Part model, mm, in its own coordinate system. Give positions to 0.01 mm unless a question says otherwise; leave off trailing zeros. Write each loop counter-clockwise with the first axis right and the second up, starting at its lowest first coordinate (ties: lowest second). Pieces come first, ordered by that corner, then holes. Notation, with made-up numbers: M -13,84.25 L 6,84.25 A18 ccw 6,109.25 Z; hole C 36.5,29.25 d4. An arc over 180 degrees is marked long. Use CSV: the item, a comma, the result in double quotes. Start each with the question number.
1. Mould opens along Z. For faces 1 (the face through (66.183, 1.479, 68.153)), 2 (the face through (57, 3, 57)), 3 (the face through (83.29, 1.48, 6.55)) say: pulls with the +Z half, pulls with the -Z half, needs draft (parallel to the pull), parting line crosses it, or undercut.
2. Band-saw the part on D-D, the plane y = 0.8. Count the separate pieces of the cut face and the enclosed holes in it, then the cut area to 3 significant figures.
3. Drop flat-ended pins along their axis: pin 1 Ø4 at (x, z) = (0, 89) entering from -Y; pin 2 Ø2 at (x, z) = (6.93, 85) entering from +Y; pin 3 Ø1.5 at (x, y) = (12, 1.5) entering from +Z; pin 4 Ø1.5 at (y, z) = (0.5, 67) entering from +X. Give the stop position or say it passes through.
4. Band-saw the part on B-B, the plane x = 0. List the corners of the cut face in (y, z), then the cut area to 3 significant figures.
5. Band-saw the part on A-A, the plane z = 0. List the corners of the cut face in (x, y), then the cut area to 3 significant figures.
6. Band-saw the part on C-C, the plane z = 89. List the corners of the cut face in (x, y), then the cut area to 3 significant figures.
7. Drill centre lines: line 1 along X through (y, z) = (0.9, 0); line 2 along Z through (x, y) = (-1, 2.7); line 3 along Z through (x, y) = (85, 1.1). Where is each one in solid material? Low to high. Write a range as from..to.
from build123d import *

# Parameters (mm, degrees)
SKETCH_1_R      = 1.75
EXTRUDE_1_DEPTH = 3


with BuildPart() as part:
    # 草图1 → 凸台-拉伸1 (new body)
    with BuildSketch(Plane(origin=(0, 0, 0), x_dir=(1, 0, 0), z_dir=(0, 1, 0))):
        with BuildLine():
            Line((-19.411428383, -72.444436972), (-24.587809285, -91.762953497))
            ThreePointArc((-24.587809285, -91.762953497), (67.175144213, -67.175144213), (91.762953497, 24.587809285))
            Line((91.762953497, 24.587809285), (72.444436972, 19.411428383))
            ThreePointArc((72.444436972, 19.411428383), (53.033008589, -53.033008589), (-19.411428383, -72.444436972))
        make_face()
        with Locations(Location((0, -89, 0), (0, 0, 270))):
            Circle(SKETCH_1_R, mode=Mode.SUBTRACT)
        with Locations(Location((0, -81, 0), (0, 0, 270))):
            Circle(SKETCH_1_R, mode=Mode.SUBTRACT)
        with Locations(Location((-6.92820323, -85, 0), (0, 0, 270))):
            Circle(SKETCH_1_R, mode=Mode.SUBTRACT)
        with Locations(Location((6.92820323, -85, 0), (0, 0, 270))):
            Circle(SKETCH_1_R, mode=Mode.SUBTRACT)
        with Locations(Location((85, -6.92820323, 0), (0, 0, 270))):
            Circle(SKETCH_1_R, mode=Mode.SUBTRACT)
        with Locations(Location((81, 0, 0), (0, 0, 270))):
            Circle(SKETCH_1_R, mode=Mode.SUBTRACT)
        with Locations(Location((85, 6.92820323, 0), (0, 0, 270))):
            Circle(SKETCH_1_R, mode=Mode.SUBTRACT)
        with Locations(Location((89, 0, 0), (0, 0, 270))):
            Circle(SKETCH_1_R, mode=Mode.SUBTRACT)
    extrude(amount=EXTRUDE_1_DEPTH)


solid = part.part
Output:
1,face 1,"parting line crosses it"
1,face 2,"needs draft"
1,face 3,"undercut"
2,separate pieces,"1"
2,enclosed holes,"8"
2,area,"3,480 mm²"
3,pin 1,"stops at y = 0"
3,pin 2,"passes through"
3,pin 3,"stops at z = 94.33"
3,pin 4,"stops at x = 68.09"
4,outline,"M 0,75 L 3,75 L 3,79.25 L 0,79.25 Z; M 0,82.75 L 3,82.75 L 3,87.25 L 0,87.25 Z; M 0,90.75 L 3,90.75 L 3,95 L 0,95 Z"
4,area,"39.0 mm²"
5,outline,"M 75,0 L 79.25,0 L 79.25,3 L 75,3 Z; M 82.75,0 L 87.25,0 L 87.25,3 L 82.75,3 Z; M 90.75,0 L 95,0 L 95,3 L 90.75,3 Z"
5,area,"39.0 mm²"
6,outline,"M -23.85,0 L -1.75,0 L -1.75,3 L -23.85,3 Z; M 1.75,0 L 33.23,0 L 33.23,3 L 1.75,3 Z"
6,area,"161 mm²"
7,line 1,"x = 75..79.25, 82.75..87.25, 90.75..95"
7,line 2,"z = 74.99..79.56, 82.44..87.56, 90.44..94.99"
7,line 3,"z = -22.78..-8.68, -5.18..5.18, 8.68..42.43"
